CAD build for the part. Positions are in the model's coordinates, mm. Face numbers are marked on the shaded views. A direction names the side the tool comes from. Give positions to 0.01 mm unless a question says otherwise; leave off trailing zeros. Write each loop counter-clockwise with the first axis right and the second up, starting at its lowest first coordinate (ties: lowest second). Pieces come first, ordered by that corner, then holes. Notation, with made-up numbers: (60.5, 59.25) -> (98.5, 59.25) arc R23 cw to (98.5, 79.25) -> close; hole circle Ø2 at (43.25, -19.75). An arc over 180 degrees is marked (long way). Answer in a Markdown table with one row per item. Add a question column.
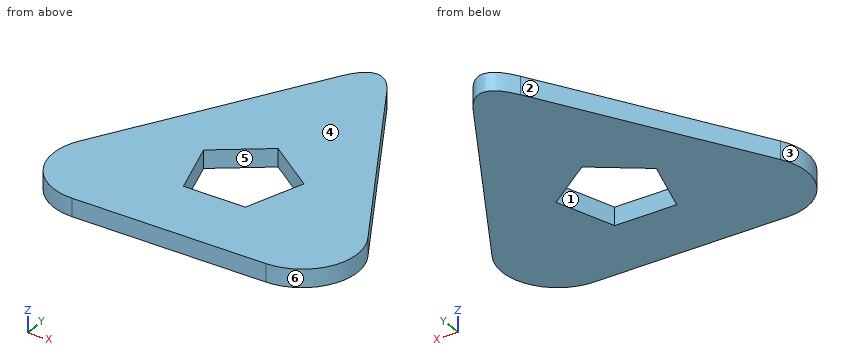
```python
from build123d import *

# Parameters (mm, degrees)
F1_DEPTH    = 1.65862
F2_T1_DEPTH = 23.6556652561
F3_R        = 5.08
F4_R        = 5.08
F6_DEPTH    = 25.4


# Not quite as in the source:
# - a fillet or chamfer that OpenCascade refuses, or shapes differently, is made with other operations: its cross-section is extruded or revolved along the edge and cut away or added


with BuildPart() as f1:
    # F0 (on Top) → F1 (new body)
    with BuildSketch(Plane.XY):
        Polygon((17.8223861725, -10.2897594543), (0, 20.5795189086), (-17.8223861725, -10.2897594543), align=None)
    extrude(amount=F1_DEPTH)

    # F2: fillet of radius 2.54 on 1 edges, made by hand

    # F2_s2 → F2_t1 (cut)
    with BuildSketch(Plane.XY.offset(-10.9985226281)):
        with BuildLine():
            add(Edge.make_bspline(
                [(2.1997045256, 16.7695189086), (0, 20.5795189086), (-2.1997045256, 16.7695189086)],
                knots=[0, 0, 0, 1, 1, 1], degree=2, weights=[1, 1, 1]))
            Line((-2.1997045256, 16.7695189086), (0, 20.5795189086))
            Line((0, 20.5795189086), (2.1997045256, 16.7695189086))
        make_face()
    extrude(amount=F2_T1_DEPTH, mode=Mode.SUBTRACT)

    # F3
    f3_edges = [f1.edges().sort_by_distance(p)[0] for p in [
        (-17.822386, -10.289759, 0.82931),
    ]]
    fillet(f3_edges, radius=F3_R)

    # F4
    f4_edges = [f1.edges().sort_by_distance(p)[0] for p in [
        (17.822386, -10.289759, 0.82931),
    ]]
    fillet(f4_edges, radius=F4_R)

    # F5 (on face) → F6 (cut)
    with BuildSketch(Plane.XY.offset(1.65862)):
        Polygon((4.6700308471, 1.5173850042), (0, 4.9103610218), (-4.6700308471, 1.5173850042), (-2.886237792, -3.9725655151), (2.886237792, -3.9725655151), align=None)
    extrude(amount=-F6_DEPTH, mode=Mode.SUBTRACT)


solid = f1.part
```
Item 1: Drop flat-ended pins along their axis: pin 1 Ø10 at (x, y) = (-6.5, -3) entering from -Z; pin 2 Ø0.8 at (x, z) = (-0.5, 0.5) entering from +Y. Give the stop position or say it passes through.
Item 2: Mould opens along Y. For the marked faces 1, 2, 3 and 4 say: released by +Y, released by -Y, zero draft, split by the parting line, or undercut.
Item 3: Slice it at A-A, the plane y = 4. List the corners of the cut face in (x, z).
Item 4: Slice it at D-D, the plane y = -7.25. List the corners of the cut face in (x, z).
Item 5: Slice it at C-C, the plane x = -6.5. List the corners of the cut face in (y, z), then the cut area to 3 significant figures.
Item 6: Which spindle directions (+Z, -Z, +X, -X, +Y, -Y) get a long thin tool onto all of the face, cutting with end or side? Do the marked faces 5 and 6. Say none if no direction does.
Item 7: Slice it at B-B, the plane y = -0.25. List the corners of the cut face in (x, z), then the cut area to 3 significant figures.
Item 8: Probe L1, parallel to X at y = 12.5, z = 0.75; L2, parallel to X at y = 1.5, z = 0.2; L3, parallel to X at y = -0.25, z = 0.25. List the from-to ranges inside material, lowest first. Write a range as from..to.
Answer key:
| question | item | result |
|---|---|---|
| 1 | pin 1 | stops at z = 0 |
| 1 | pin 2 | stops at y = 18.67 |
| 2 | face 1 | undercut |
| 2 | face 2 | released by +Y |
| 2 | face 3 | split by the parting line |
| 2 | face 4 | zero draft |
| 3 | outline | (-9.57, 0) -> (-1.25, 0) -> (-1.25, 1.66) -> (-9.57, 1.66) -> close; (1.25, 0) -> (9.57, 0) -> (9.57, 1.66) -> (1.25, 1.66) -> close |
| 4 | outline | (-13.68, 0) -> (13.68, 0) -> (13.68, 1.66) -> (-13.68, 1.66) -> close |
| 5 | outline | (-10.29, 0) -> (9.32, 0) -> (9.32, 1.66) -> (-10.29, 1.66) -> close |
| 5 | area | 32.5 mm² |
| 6 | face 5 | +Z, -Z |
| 6 | face 6 | +Z, -Z, +X |
| 7 | outline | (-12.03, 0) -> (-4.1, 0) -> (-4.1, 1.66) -> (-12.03, 1.66) -> close; (4.1, 0) -> (12.03, 0) -> (12.03, 1.66) -> (4.1, 1.66) -> close |
| 7 | area | 26.3 mm² |
| 8 | L1 | x = -4.66..4.66 |
| 8 | L2 | x = -11.02..-4.66, 4.66..11.02 |
| 8 | L3 | x = -12.03..-4.1, 4.1..12.03 |
